```python
from build123d import *

# Parameters (mm, degrees)
BOSS_EXTRUDE1_DEPTH = 3.556


with BuildPart() as part:
    # Sketch1 → Boss-Extrude1 (new body)
    with BuildSketch(Plane.XY):
        with BuildLine():
            Line((-161.499532604, 280.561645896), (-161.499532604, 356.788581407))
            Line((-161.499532604, 356.788581407), (-301.19953221, 356.788581407))
            Line((-301.19953221, 356.788581407), (-301.19953221, 280.561645896))
            Line((-301.19953221, 280.561645896), (-282.884212388, 248.838581407))
            ThreePointArc((-282.884212388, 248.838581407), (-268.938644504, 234.893013523), (-249.888644504, 229.788581407))
            Line((-249.888644504, 229.788581407), (-212.81042031, 229.788581407))
            ThreePointArc((-212.81042031, 229.788581407), (-193.76042031, 234.893013523), (-179.814852426, 248.838581407))
            Line((-179.814852426, 248.838581407), (-161.499532604, 280.561645896))
        make_face()
    extrude(amount=-BOSS_EXTRUDE1_DEPTH)


solid = part.part
```
Here's how the part is built. I have some questions about the finished solid (model axes, mm). Round coordinates to 2 decimals unless told otherwise and drop trailing zeros. Write each loop counter-clockwise with the first axis right and the second up, starting at its lowest first coordinate (ties: lowest second). Pieces come first, ordered by that corner, then holes.
Q1. Please list where these lines run through material, in increasing order: probe 1 along X at (y, z) = (276.5, -2.3); probe 2 along Y at (x, z) = (-173, -1.05); probe 3 along X at (y, z) = (253.5, -2.45).
Q2. If we section it at B-B on y = 278.5: Write out the boundary of the cut face in (x, z).
Q3. If we section it at A-A on z = -2.1: Write out the boundary of the cut face in (x, y).
Q4. Will this pin go through, and if not, where does the flat tip stop? P1, Ø4, axis at x = -256.5, y = 304, coming from the +Z side.
Answer below:
1. probe 1: x = -298.85 to -163.84
1. probe 2: y = 260.64 to 356.79
1. probe 3: x = -285.58 to -177.12
2. outline: (-300.01, -3.56) - (-162.69, -3.56) - (-162.69, 0) - (-300.01, 0) - close
3. outline: (-301.2, 280.56) - (-282.88, 248.84) arc R38.1 ccw to (-249.89, 229.79) - (-212.81, 229.79) arc R38.1 ccw to (-179.81, 248.84) - (-161.5, 280.56) - (-161.5, 356.79) - (-301.2, 356.79) - close
4. P1: stops at z = 0
